```python
from build123d import *

# Parameters (mm, degrees)
SKETCH1_W               = 50.8
SKETCH1_H               = 25.4
BOSS_EXTRUDE1_DEPTH     = 4.318
SKETCH2_W               = 6.35
SKETCH2_H               = 25.4
BOSS_EXTRUDE2_DEPTH     = 27.432
SKETCH4_R               = 2.413
CUT_EXTRUDE1_DEPTH      = 4.318
CUT_EXTRUDE2_DEPTH      = 57.081681501
CUT_EXTRUDE2_DEPTH_BACK = 57.081681501
SKETCH5_R               = 2.413


with BuildPart() as part:
    # Sketch1 → Boss-Extrude1 (new body)
    with BuildSketch(Plane.XY):
        Rectangle(SKETCH1_W, SKETCH1_H)
    extrude(amount=BOSS_EXTRUDE1_DEPTH)

    # Sketch2 → Boss-Extrude2 (add)
    with BuildSketch(Plane.XY.offset(4.318)):
        with Locations((-22.225, 0)):
            Rectangle(SKETCH2_W, SKETCH2_H)
        with Locations((22.225, 0)):
            Rectangle(SKETCH2_W, SKETCH2_H)
    extrude(amount=BOSS_EXTRUDE2_DEPTH)

    # Sketch4 → Cut-Extrude1 (cut)
    with BuildSketch(Plane(origin=(0, 0, 0), x_dir=(-1, 0, 0), z_dir=(0, 0, -1))):
        with Locations((-9.525, 0)):
            Circle(SKETCH4_R)
        with Locations((9.525, 0)):
            Circle(SKETCH4_R)
    extrude(amount=-CUT_EXTRUDE1_DEPTH, mode=Mode.SUBTRACT)

    # Sketch5 → Cut-Extrude2 (cut, two sides: drawn at the far end of the back side and taken through both)
    with BuildSketch(Plane(origin=(-19.05, 0, 0), x_dir=(0, 0, -1), z_dir=(1, 0, 0)).offset(-CUT_EXTRUDE2_DEPTH_BACK)):
        with Locations((-18.034, 0)):
            Circle(SKETCH5_R)
    extrude(amount=CUT_EXTRUDE2_DEPTH + CUT_EXTRUDE2_DEPTH_BACK, mode=Mode.SUBTRACT)


solid = part.part
```
Model file for the job. Use its own axes, mm. A direction names the side the tool comes from. Coordinates: 2 decimals unless noted, no trailing zeros. Order: outer loops, then holes, each group sorted by start corner. A loop starts at its lowest first (then second) coordinate and runs counter-clockwise, first axis right, second up. Notation, with made-up numbers: M -32.5,60 L -16.5,60 A15 cw -16.5,80 Z; hole C 40,-13 d3. An arc over 180 degrees is marked long. Answer as CSV lines item,"result".
(1) Band-saw the part on D-D, the plane y = 3.75. List the corners of the cut face in (x, z).
Geometry says:
outline,"M -25.4,0 L 25.4,0 L 25.4,31.75 L 19.05,31.75 L 19.05,4.32 L -19.05,4.32 L -19.05,31.75 L -25.4,31.75 Z"
(2) Band-saw the part on C-C, the plane x = 9. List the corners of the cut face in (y, z), then the cut area to 3 significant figures.
Geometry says:
outline,"M -12.7,0 L -2.36,0 L -2.36,4.32 L -12.7,4.32 Z; M 2.36,0 L 12.7,0 L 12.7,4.32 L 2.36,4.32 Z"
area,"89.3 mm2"
(3) Flat gauge pin, fed straight in: pin 1 (6.5 mm diameter, centred on x = 9.525, y = 0, fed in from +Z). Where does the tip first touch, or does it go through?
Geometry says:
pin 1,"stops at z = 4.32"
(4) Band-saw the part on B-B, the plane y = 0. List the corners of the cut face in (x, z).
Geometry says:
outline,"M -25.4,0 L -11.94,0 L -11.94,4.32 L -19.05,4.32 L -19.05,15.62 L -25.4,15.62 Z; M -25.4,20.45 L -19.05,20.45 L -19.05,31.75 L -25.4,31.75 Z; M -7.11,0 L 7.11,0 L 7.11,4.32 L -7.11,4.32 Z; M 11.94,0 L 25.4,0 L 25.4,15.62 L 19.05,15.62 L 19.05,4.32 L 11.94,4.32 Z; M 19.05,20.45 L 25.4,20.45 L 25.4,31.75 L 19.05,31.75 Z"
(5) 3-axis set-ups, long thin cutter, end or side, ignore diameter. For faces 1 (the flat face through (19.05, 3, 18)), 2 (the flat face through (0, -12.7, 4)): which of +Z, -Z, +X, -X, +Y, -Y reach the whole face in a straight line?
Geometry says:
face 1,"+Z, +Y, -Y"
face 2,"+Z, -Z, +X, -X, -Y"
(6) Wall check: line 1 along X through (y, z) = (11, 11.5); line 2 along Z through (x, y) = (21.75, 0); line 3 along Z through (x, y) = (-7, 10.75). Give the ranges that are in metal, low to high.
Geometry says:
line 1,"x = -25.4 to -19.05, 19.05 to 25.4"
line 2,"z = 0 to 15.62, 20.45 to 31.75"
line 3,"z = 0 to 4.32"
(7) Band-saw the part on A-A, the plane z = 14.5. List the corners of the cut face in (x, y).
Geometry says:
outline,"M -25.4,-12.7 L -19.05,-12.7 L -19.05,12.7 L -25.4,12.7 Z; M 19.05,-12.7 L 25.4,-12.7 L 25.4,12.7 L 19.05,12.7 Z"
(8) Pull direction Y, two halves, no side cores. Call faces 3 (the flat face through (0, 12.7, 4)), 4 (the flat face through (-25.4, 3, 16)), 5 (the cylindrical face through (-22.269, 0.106, 20.445)): +Y half, -Y half, draft (parallel to the pull), parting line (faces both ways), or undercut.
Geometry says:
face 3,"+Y half"
face 4,"draft"
face 5,"undercut"
